Geometry check sheet. Reference: the model listing, model coordinates, mm. A direction names the side the tool comes from. Round coordinates to 2 decimals unless told otherwise and drop trailing zeros. Write each loop counter-clockwise with the first axis right and the second up, starting at its lowest first coordinate (ties: lowest second). Pieces come first, ordered by that corner, then holes. Notation, with made-up numbers: (16.5, 64) - (42.5, 64) arc R15 ccw to (42.5, 73) - close; hole circle Ø6 at (19.25, -34). An arc over 180 degrees is marked (long way). One line per question, with ' | ' between items. Start each with the question number.
from build123d import *

# Parameters (mm, degrees)
F0_R     = 4
F1_DEPTH = 32.5
F3_DEPTH = 7


# Not quite as in the source:
# - a pattern or mirror of a feature is missing from the dataset's text; its kind, count and spacing are read off the source's solid


with BuildPart() as f1:
    # F0 (on Front) → F1 (new body, symmetric)
    with BuildSketch(Plane.XZ):
        Circle(F0_R)
    extrude(amount=F1_DEPTH, both=True)

    # F2 (on face) → F3 (cut)
    with BuildSketch(Plane.XZ.offset(32.5)):
        Polygon((0, 4.634491168), (-1, 3.8729833462), (-1, 2.8729833462), (1, 2.8729833462), (1, 3.8729833462), align=None)
    f3 = extrude(amount=-F3_DEPTH, mode=Mode.SUBTRACT)

    # F3_copies: F3 across plane
    add(f3.mirror(Plane.ZX), mode=Mode.SUBTRACT)


solid = f1.part
Q1. Section check C-C, the plane y = -2. Record the cut outline in (x, z), then the cut area to 3 significant figures.
Q2. Section check A-A, the plane x = 0. Record the cut outline in (y, z).
Q3. Section check B-B, the plane y = 27.5. Record the cut outline in (x, z).
Q4. Set-up check for faces 1 (the flat face through (-1, -29, 3.4)), 2 (the flat face through (0, 29, 2.873)), 3 (the flat face through (0, 32.5, 0)): record each of +Z, -Z, +X, -X, +Y, -Y from which the full face is reachable in a straight line by a thin tool's end or side.
Q5. Thickness scan on line 1 (Z direction, x = 0, y = 28); line 2 (Z direction, x = -0.25, y = 3); line 3 (X direction, y = 25.5, z = -2). Record the ranges inside material, lowest first.
Q6. Draft check along X on faces 4 (the flat face through (0, 25.5, 3.4)), 5 (the flat face through (0, -32.5, 0)), 6 (the cylindrical face through (-0.867, -0.455, -3.905)). Enter one of: pulls with the +X half, pulls with the -X half, needs draft (parallel to the pull), parting line crosses it, or undercut.
Q7. Section check D-D, the plane x = -3. Record the cut outline in (y, z), then the cut area to 3 significant figures.
Q8. Go/stop test with flat-tipped pins: P1, Ø2, axis at x = -0.5, y = 28.5, coming from the +Z side; P2, Ø1.1, axis at y = -30, z = 3, coming from the -X side; P3, Ø0.8, axis at y = 28, z = 3, coming from the +X side. Record where each tip stops, or that it passes through.
Result sheet:
1) outline: circle Ø8 at (0, 0) | area: 50.3 mm²
2) outline: (-32.5, -4) - (32.5, -4) - (32.5, 2.87) - (25.5, 2.87) - (25.5, 4) - (-25.5, 4) - (-25.5, 2.87) - (-32.5, 2.87) - close
3) outline: (-1, 2.87) - (-1, 3.87) arc R4 ccw (long way) to (1, 3.87) - (1, 2.87) - close
4) face 1: +Z, -Y | face 2: +Z, +Y | face 3: +Z, -Z, +X, -X, +Y
5) line 1: -4 to 2.87 | line 2: -3.99 to 3.99 | line 3: -3.46 to 3.46
6) face 4: undercut | face 5: needs draft | face 6: parting line crosses it
7) outline: (-32.5, -2.65) - (32.5, -2.65) - (32.5, 2.65) - (-32.5, 2.65) - close | area: 344 mm²
8) P1: z = 3.87 | P2: x = -3.16 | P3: x = 3.04
